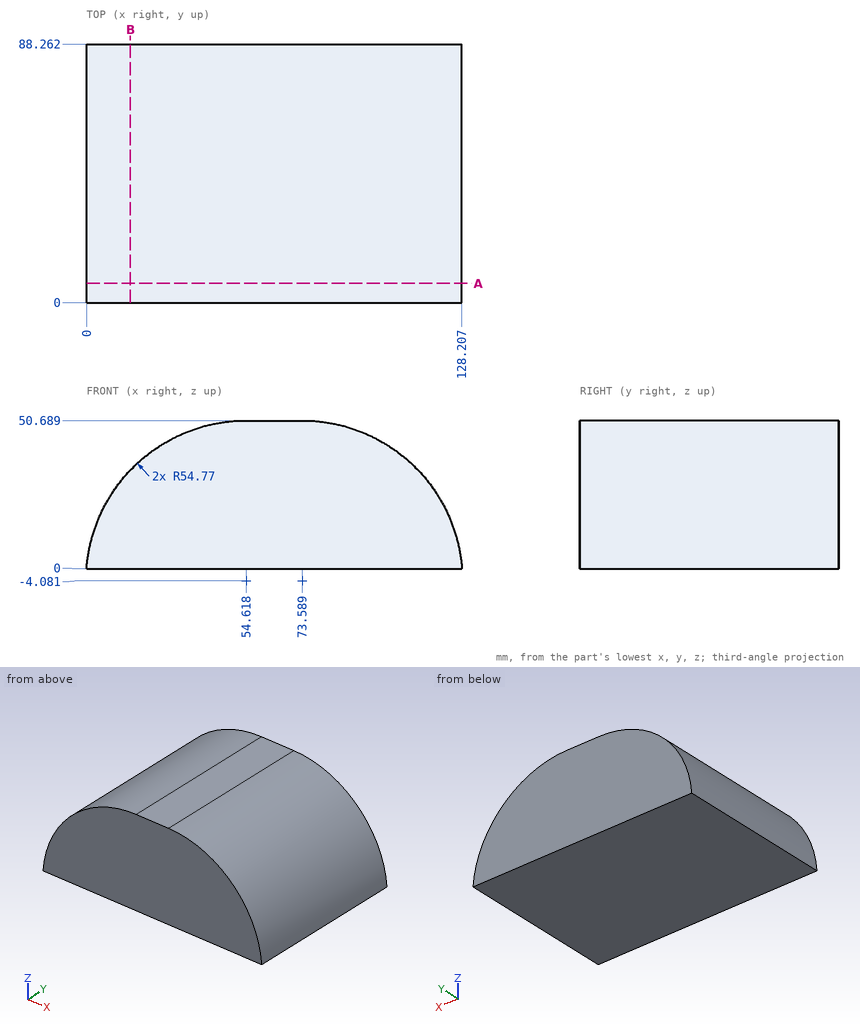
Study the drawing (mm; zero at the part's minimum x, y, z) and answer. Give positions to 0.01 mm unless a question says otherwise; leave off trailing zeros. Write each loop counter-clockwise with the first axis right and the second up, starting at its lowest first coordinate (ties: lowest second). Pieces come first, ordered by that corner, then holes. Notation, with made-up numbers: (89, 41) -> (134, 41) arc R15 ccw to (134, 67) -> close; hole circle Ø6 at (-7, -14.75). An arc over 180 degrees is marked (long way). Write item = value, one per line. Start each with the question number.
1) The part is cut by section B-B, the plane x = 15. Determine the outline of the cut face in (y, z).
2) Straight lines are drawn through the part: line 1 along X through (y, z) = (45.5, 9) (1 decimal); line 2 along X through (y, z) = (77, 8); line 3 along Z through (x, y) = (76, 40). For each, find the intervals that lie inside material, in ascending order.
3) Each of these flat-tipped pins is pushed along its axis until it touches: pin 1 (1.5 mm diameter, centred on y = 44.5, z = 32.5, fed in from -X) (1 decimal); pin 2 (10 mm diameter, centred on y = 48.5, z = 18, fed in from +X); pin 3 (1 mm diameter, centred on x = 25, y = 10, fed in from +Z); pin 4 (12 mm diameter, centred on x = 94.5, y = 65, fed in from -Z). Where does it stop, or does it pass through?
4) The part is cut by section A-A, the plane y = 6.5. Determine the outline of the cut face in (x, z).
Solutions:
q1.outline = (0, 0) -> (88.26, 0) -> (88.26, 33.74) -> (0, 33.74) -> close
q2.line_1 = 1.4 to 126.8
q2.line_2 = 1.2 to 127.01
q2.line_3 = 0 to 50.64
q3.pin_1 = 13.2
q3.pin_2 = 125.63
q3.pin_3 = 42.31
q3.pin_4 = 0
q4.outline = (0, 0) -> (128.21, 0) arc R54.77 ccw to (73.59, 50.69) -> (54.62, 50.69) arc R54.77 ccw to start
